Can you work these out from the drawing? Everything is in mm from the part's minimum corner. A direction names the side the tool comes from. Round coordinates to 2 decimals unless told otherwise and drop trailing zeros. Order: outer loops, then holes, each group sorted by start corner. A loop starts at its lowest first (then second) coordinate and runs counter-clockwise, first axis right, second up. Notation, with made-up numbers: (-22.5, 35.5) -> (9.5, 35.5) arc R25 ccw to (9.5, 50.5) -> close; hole circle Ø3 at (-10, -11). An arc over 180 degrees is marked (long way). One line per item, written item: value.
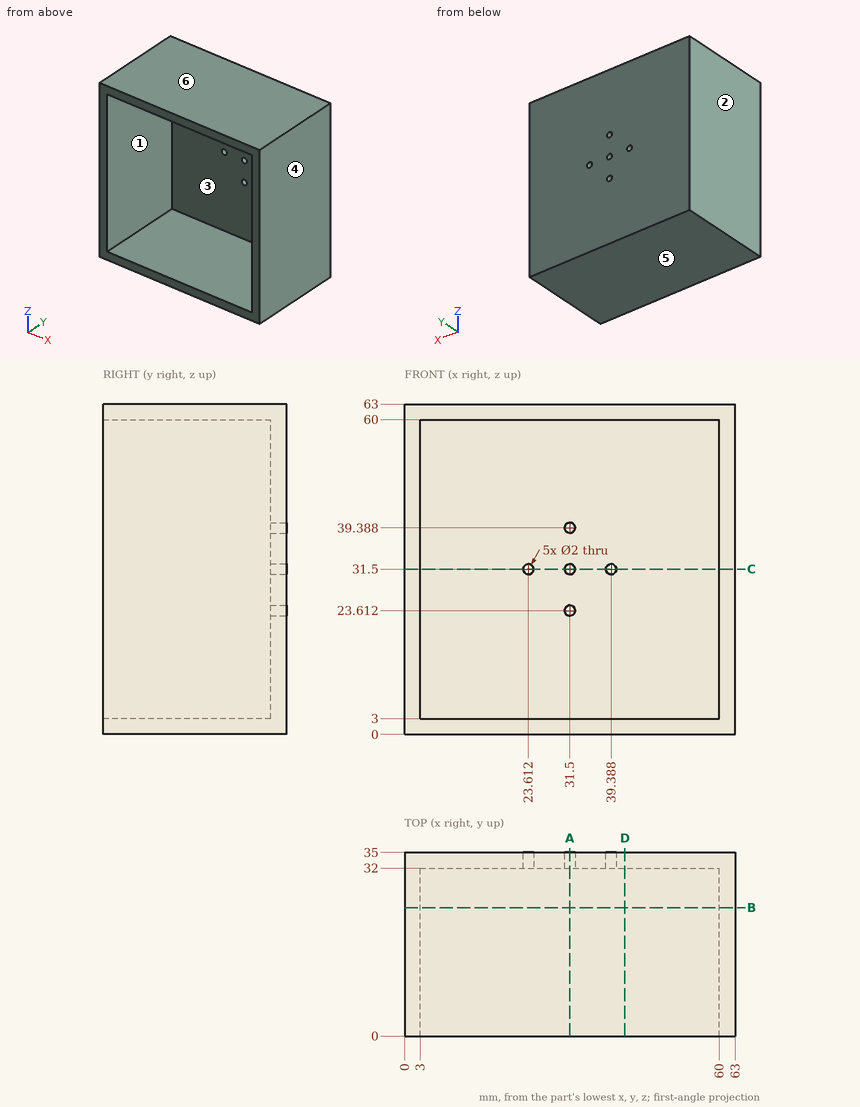
Q1. On a 3-axis mill with a long thin cutter (end or side, diameter ignored), from which of +Z, -Z, +X, -X, +Y, -Y can I reach the whole of each face in a straight line? I mean the marked faces 1 and 2. Say none if no direction works.
Answers below:
face 1: -Y
face 2: +Z, -Z, -X, +Y, -Y
Q2. I want a section at D-D on x = 42. List the corners of the cut face in (y, z) for me.
Answers below:
outline: (0, 0) -> (35, 0) -> (35, 63) -> (0, 63) -> (0, 60) -> (32, 60) -> (32, 3) -> (0, 3) -> close
Q3. I want a section at B-B on y = 24.5. List the corners of the cut face in (x, z) for me.
Answers below:
outline: (0, 0) -> (63, 0) -> (63, 63) -> (0, 63) -> close; hole (3, 3) -> (60, 3) -> (60, 60) -> (3, 60) -> close
Q4. Will these pins go through, and if not, where does the flat tip stop? pin 1 Ø17 at (x, z) = (27, 40) entering from -Y; pin 2 Ø1.8 at (x, z) = (31.5, 39.39) entering from -Y.
Answers below:
pin 1: y = 32
pin 2: through
Q5. Please list where these lines run through material, in increasing order: line 1 along X through (y, z) = (12.5, 35.5); line 2 along X through (y, z) = (33.15, 31.5).
Answers below:
line 1: 0 to 3, 60 to 63
line 2: 0 to 22.61, 24.61 to 30.5, 32.5 to 38.39, 40.39 to 63
Q6. We'd pull the mould along Z, two halves only. Please class the marked faces 3, 4, 5 and 6: released by +Z, released by -Z, zero draft, split by the parting line, or undercut.
Answers below:
face 3: undercut
face 4: zero draft
face 5: released by -Z
face 6: released by +Z
Q7. I want a section at A-A on x = 31.5. List the corners of the cut face in (y, z) for me, plus the area to 3 significant figures.
Answers below:
outline: (0, 0) -> (35, 0) -> (35, 22.61) -> (32, 22.61) -> (32, 3) -> (0, 3) -> close; (0, 60) -> (32, 60) -> (32, 40.39) -> (35, 40.39) -> (35, 63) -> (0, 63) -> close; (32, 24.61) -> (35, 24.61) -> (35, 30.5) -> (32, 30.5) -> close; (32, 32.5) -> (35, 32.5) -> (35, 38.39) -> (32, 38.39) -> close
area: 363 mm^2
Q8. I want a section at C-C on z = 31.5. List the corners of the cut face in (x, y) for me.
Answers below:
outline: (0, 0) -> (3, 0) -> (3, 32) -> (22.61, 32) -> (22.61, 35) -> (0, 35) -> close; (24.61, 32) -> (30.5, 32) -> (30.5, 35) -> (24.61, 35) -> close; (32.5, 32) -> (38.39, 32) -> (38.39, 35) -> (32.5, 35) -> close; (40.39, 32) -> (60, 32) -> (60, 0) -> (63, 0) -> (63, 35) -> (40.39, 35) -> close
